```python
from build123d import *

# Parameters (mm, degrees)
F0_W     = 20
F0_H     = 20
F1_DEPTH = 40
F2_W     = 20
F2_H     = 10
F3_DEPTH = 25
F4_R     = 6.5
F5_DEPTH = 40.001


with BuildPart() as f1:
    # F0 (on Top) → F1 (new body)
    with BuildSketch(Plane.XY):
        with Locations((-97.988032, 0)):
            Rectangle(F0_W, F0_H)
    extrude(amount=F1_DEPTH)

    # F2 (on face) → F3 (join)
    with BuildSketch(Plane.YZ.offset(-87.988032)):
        with Locations((0, 35)):
            Rectangle(F2_W, F2_H)
    extrude(amount=F3_DEPTH)

    # F4 (on face) → F5 (cut, through all)
    with BuildSketch(Plane.XY.offset(40)):
        with Locations((-74.988032, 0)):
            Circle(F4_R)
    extrude(amount=-F5_DEPTH, mode=Mode.SUBTRACT)


solid = f1.part
```
The model under review builds one solid part; all positions refer to its coordinate system, in mm. A direction names the side the tool comes from. Give positions to 0.01 mm unless a question says otherwise; leave off trailing zeros. Write each loop counter-clockwise with the first axis right and the second up, starting at its lowest first coordinate (ties: lowest second). Pieces come first, ordered by that corner, then holes. Notation, with made-up numbers: M 78,-11 L 109,-11 A16 cw 109,3 Z; hole C -5,72.5 d8. An arc over 180 degrees is marked long. Write each question's results on one line, items separated by ' | '. Start each with the question number.
1. Mouldability with a two-part tool opening along Y and no side actions: class faces 1 (the flat face through (-96, 10, 24)), 2 (the flat face through (-87.988, 0, 15)), 3 (the cylindrical face through (-81.48, 0.29, 35.07)), 4 (the flat face through (-96, -10, 24)) as released by +Y, released by -Y, zero draft, split by the parting line, or undercut.
2. We need section A-A (y = 0). Write out the cut boundary in (x, z), and give its area (3 significant figures).
3. For probe 1 along Z at (x, y) = (-85.5, -3.5); probe 2 along X at (y, z) = (-6.75, 29.5); probe 3 along Y at (x, z) = (-69, 35.5), list the stretches that pass through material, from the lowest coordinate up. Write a range as [from, to].
4. For faces 5 (the flat face through (-62.988, 0, 35)), 6 (the flat face through (-81.2, -2.4, 30)), list the 3-axis set-ups (+Z, -Z, +X, -X, +Y, -Y) from which the entire face can be reached by the end or side of a thin tool; tool diameter is ignored.
5. We need section D-D (y = -5.5). Write out the cut boundary in (x, z), and give its area (3 significant figures).
6. Insertion check: pin 1 Ø4 at (x, y) = (-79.5, 4) entering from -Z; pin 2 Ø4 at (x, z) = (-87.5, 14) entering from -Y. Each pin has a flat end and moves straight along its axis. Give the tip position at first contact, or say it passes through.
7. We need section B-B (x = -79). Write out the cut boundary in (y, z).
8. We need section C-C (z = 28.5). Write out the cut boundary in (x, y).
Results found:
1) face 1: released by +Y | face 2: zero draft | face 3: undercut | face 4: released by -Y
2) outline: M -107.99,0 L -87.99,0 L -87.99,30 L -81.49,30 L -81.49,40 L -107.99,40 Z; M -68.49,30 L -62.99,30 L -62.99,40 L -68.49,40 Z | area: 920 mm^2
3) probe 1: z = [30, 40] | probe 2: x = [-107.99, -87.99] | probe 3: y = [-10, -2.53], [2.53, 10]
4) face 5: +Z, -Z, +X, +Y, -Y | face 6: -Z, +X, +Y, -Y
5) outline: M -107.99,0 L -87.99,0 L -87.99,30 L -78.45,30 L -78.45,40 L -107.99,40 Z; M -71.52,30 L -62.99,30 L -62.99,40 L -71.52,40 Z | area: 981 mm^2
6) pin 1: stops at z = 30 | pin 2: stops at y = -10
7) outline: M -10,30 L -5.11,30 L -5.11,40 L -10,40 Z; M 5.11,30 L 10,30 L 10,40 L 5.11,40 Z
8) outline: M -107.99,-10 L -87.99,-10 L -87.99,10 L -107.99,10 Z
